Could you check a few things on this model? Use its own coordinates, in mm. A direction names the side the tool comes from. Give positions to 0.01 mm unless a question says otherwise; leave off trailing zeros. Loops run counter-clockwise (first coordinate to the right, second up) from the corner with the lowest first, then second, coordinate; pieces in that order, holes last. Notation, with made-up numbers: (58, 13.5) -> (77, 13.5) arc R25 cw to (77, 31.5) -> close; hole circle Ø11 at (11, 47). An arc over 180 degrees is marked (long way). Put each result on its own line as item: value.
```python
from build123d import *

# Parameters (mm, degrees)
F1_DEPTH    = 180
F2_R        = 5
F3_T1_DEPTH = 191.1494898741


# Not quite as in the source:
# - a fillet or chamfer that OpenCascade refuses, or shapes differently, is made with other operations: its cross-section is extruded or revolved along the edge and cut away or added


with BuildPart() as f1:
    # F0 (on Top) → F1 (new body)
    with BuildSketch(Plane.XY):
        with BuildLine():
            ThreePointArc((14.1226732436, -15.5418821401), (0.1645874713, -20.9993550131), (-13.8773267564, -15.7613388421))
            Line((-13.8773267564, -15.7613388421), (-12.7134246975, -29.6120676683))
            Line((-12.7134246975, -29.6120676683), (-6.7134246975, -29.6071426253))
            Line((-6.7134246975, -29.6071426253), (-6.7134246975, -23.6071426253))
            Line((-6.7134246975, -23.6071426253), (4.2865298223, -23.6563930556))
            Line((4.2865298223, -23.6563930556), (4.2865298223, -29.6071426253))
            Line((4.2865298223, -29.6071426253), (6.2865237583, -29.6120676683))
            Line((6.2865237583, -29.6120676683), (6.2751961593, -34.2120537211))
            Line((6.2751961593, -34.2120537211), (-12.4721404334, -34.2120676683))
            Line((-12.4721404334, -34.2120676683), (-12.4721404334, -35.7862083692))
            ThreePointArc((-12.4721404334, -35.7862083692), (-1.2161640349, -38.1355598231), (10.2751961593, -38.5418821401))
            Line((10.2751961593, -38.5418821401), (14.1226732436, -15.5418821401))
        make_face()
    extrude(amount=F1_DEPTH)

    # F2
    f2_edges = [f1.edges().sort_by_distance(p)[0] for p in [
        (10.275196, -38.541882, 90),
    ]]
    fillet(f2_edges, radius=F2_R)

    # F3: fillet of radius 3 on 1 edges, made by hand

    # F3_s2 → F3_t1 (cut)
    with BuildSketch(Plane.XY.offset(-5.5747449371)):
        with BuildLine():
            ThreePointArc((-10.3257108334, -36.3905964487), (-11.6973730961, -35.5953820953), (-12.4721404334, -34.2120676683))
            Line((-12.4721404334, -34.2120676683), (-12.4721404334, -35.7862083692))
            ThreePointArc((-12.4721404334, -35.7862083692), (-11.4014196416, -36.0972596534), (-10.3257108334, -36.3905964487))
        make_face()
    extrude(amount=F3_T1_DEPTH, mode=Mode.SUBTRACT)


solid = f1.part
```
1. If we section it at A-A (x = 0.75): List the corners of the cut face in (y, z) for me.
Recorded:
outline: (-38.34, 0) -> (-34.21, 0) -> (-34.21, 180) -> (-38.34, 180) -> close; (-23.64, 0) -> (-20.99, 0) -> (-20.99, 180) -> (-23.64, 180) -> close
2. If we section it at B-B (z = 23.5): List the corners of the cut face in (x, y) for me.
Recorded:
outline: (-13.88, -15.76) -> (-12.71, -29.61) -> (-6.71, -29.61) -> (-6.71, -23.61) -> (4.29, -23.66) -> (4.29, -29.61) -> (6.29, -29.61) -> (6.28, -34.21) -> (-12.47, -34.21) arc R3 ccw to (-10.33, -36.39) arc R67.55 ccw to (5.96, -38.62) arc R5 ccw to (10.96, -34.44) -> (14.12, -15.54) arc R21 cw to start
3. Thinking about a two-plate mould opening in Y: for faces 1 (the face through (6, -27, 0)), 2 (the face through (-3, -34.212, 89)), 3 (the face through (0, -21, 89)), 4 (the face through (-13.304, -22.59, 88.74)), which applies, pulls with the +Y half, pulls with the -Y half, needs draft (parallel to the pull), parting line crosses it, or undercut?
Recorded:
face 1: needs draft
face 2: undercut
face 3: pulls with the +Y half
face 4: pulls with the -Y half
4. I'm going to push flat-ended pins straight in: pin 1 (1.8 mm diameter, centred on y = -26.5, z = 54, fed in from -X); pin 2 (5 mm diameter, centred on x = 4.5, y = -21, fed in from -Z); pin 3 (8 mm diameter, centred on x = -9.5, z = 141.5, fed in from +Y); pin 4 (1.5 mm diameter, centred on x = 3.5, z = 59, fed in from +Y). Where does each tip first touch, or does it pass through?
Recorded:
pin 1: stops at x = -13.05
pin 2: stops at z = 0
pin 3: stops at y = -16.09
pin 4: stops at y = -20.57
5. I need wall thicknesses on line 1 (Y direction, x = 2.5, z = 130.5); line 2 (X direction, y = -28.5, z = 132); line 3 (Y direction, x = -11.5, z = 118). Which ranges of each line are inside material? Lowest first, please.
Recorded:
line 1: y = -38.48 to -34.21, -23.65 to -20.85
line 2: x = -12.81 to -6.71, 4.29 to 11.96
line 3: y = -35.78 to -34.21, -29.61 to -17.57
6. For faces 5 (the face through (6, -27, 180)), 6 (the face through (4.287, -27, 89)), which set-ups out of +Z, -Z, +X, -X, +Y, -Y let a thin tool reach every point of the face, with its end or its side?
Recorded:
face 5: +Z, +X, -X, +Y, -Y
face 6: +Z, -Z
7. If we section it at C-C (y = -25.75): List the corners of the cut face in (x, z) for me.
Recorded:
outline: (-13.04, 0) -> (-6.71, 0) -> (-6.71, 180) -> (-13.04, 180) -> close; (4.29, 0) -> (12.42, 0) -> (12.42, 180) -> (4.29, 180) -> close
